Design review of the part built by this model. Coordinates are the model's own, in mm. Give positions to 0.01 mm unless a question says otherwise; leave off trailing zeros. Loops run counter-clockwise (first coordinate to the right, second up) from the corner with the lowest first, then second, coordinate; pieces in that order, holes last. Notation, with made-up numbers: M 2,-6.5 L 41,-6.5 A32 cw 41,32.5 Z; hole C 62,-34.75 d2. An arc over 180 degrees is marked long. Use one line per item in the form item = value. Start each with the question number.
from build123d import *

# Parameters (mm, degrees)
BOSS_EXTRUDE1_DEPTH     = 158.75
CUT_EXTRUDE1_DEPTH      = 160.046057271
CUT_EXTRUDE1_DEPTH_BACK = 160.046057271
SKETCH2_R               = 3.175


with BuildPart() as part:
    # Sketch1 → Boss-Extrude1 (new body)
    with BuildSketch(Plane.XY):
        Polygon((7.332348419, 0), (3.666174209, 6.35), (-3.666174209, 6.35), (-7.332348419, 0), (-3.666174209, -6.35), (3.666174209, -6.35), align=None)
    extrude(amount=BOSS_EXTRUDE1_DEPTH)

    # Sketch2 → Cut-Extrude1 (cut, two sides: drawn at the far end of the back side and taken through both)
    with BuildSketch(Plane.XY.offset(158.75).offset(-CUT_EXTRUDE1_DEPTH_BACK)):
        Circle(SKETCH2_R)
    extrude(amount=CUT_EXTRUDE1_DEPTH + CUT_EXTRUDE1_DEPTH_BACK, mode=Mode.SUBTRACT)


solid = part.part
Q1. Take a section at D-D on x = 5.75. Give the boundary of the cut face in (y, z), plus the area to 3 significant figures.
Q2. Take a section at C-C on y = -1.75. Give the boundary of the cut face in (x, z), plus the area to 3 significant figures.
Q3. Take a section at A-A on x = 0. Give the boundary of the cut face in (y, z) (3 decimals).
Q4. Take a section at B-B on z = 145.5. Give the boundary of the cut face in (x, y) (3 decimals), plus the area to 3 significant figures.
Q5. Clearance check with a flat-ended pin moving along its axis: pin 1 Ø2 at (x, y) = (1, -0.5) entering from +Z. State where the tip first meets the part, or that it passes through.
Q6. The part is to be moulded in two halves that separate along X. For faces 1 (the cylindrical face through (-0.69, -3.1, 78.26)), 2 (the flat face through (2, 3, 158.75)), 3 (the flat face through (-5.525, -3.131, 78.264)), say which applies: pulls with the +X half, pulls with the -X half, needs draft (parallel to the pull), parting line crosses it, or undercut.
Q7. Wall thickness on probe 1 along X at (y, z) = (0, 107) (3 decimals); probe 2 along Y at (x, z) = (0, 119) (3 decimals); probe 3 along X at (y, z) = (-1, 118) (3 decimals): over which ranges is each line inside the solid? List them lowest first.
Response values:
q1.outline = M -2.74,0 L 2.74,0 L 2.74,158.75 L -2.74,158.75 Z
q1.area = 870 mm^2
q2.outline = M -6.32,0 L -2.65,0 L -2.65,158.75 L -6.32,158.75 Z; M 2.65,0 L 6.32,0 L 6.32,158.75 L 2.65,158.75 Z
q2.area = 1,170 mm^2
q3.outline = M -6.35,0 L -3.175,0 L -3.175,158.75 L -6.35,158.75 Z; M 3.175,0 L 6.35,0 L 6.35,158.75 L 3.175,158.75 Z
q4.outline = M -7.332,0 L -3.666,-6.35 L 3.666,-6.35 L 7.332,0 L 3.666,6.35 L -3.666,6.35 Z; hole C 0,0 d6.35
q4.area = 108 mm^2
q5.pin_1 = through
q6.face_1 = undercut
q6.face_2 = needs draft
q6.face_3 = pulls with the -X half
q7.probe_1 = -7.332 to -3.175, 3.175 to 7.332
q7.probe_2 = -6.35 to -3.175, 3.175 to 6.35
q7.probe_3 = -6.755 to -3.013, 3.013 to 6.755
